```python
from build123d import *

# Parameters (mm, degrees)
SKETCH1_W               = 39.39
SKETCH1_H               = 10
BOSS_EXTRUDE1_DEPTH     = 20
SKETCH2_W               = 31.39
SKETCH2_H               = 10
CUT_EXTRUDE1_DEPTH      = 15
CUT_EXTRUDE2_DEPTH      = 46.294283304
CUT_EXTRUDE2_DEPTH_BACK = 46.294283304
SKETCH3_R               = 1.25
FILLET1_R               = 3
FILLET3_R               = 1
SKETCH4_W               = 20
SKETCH4_H               = 10
BOSS_EXTRUDE2_DEPTH     = 165
FILLET4_R               = 5
SKETCH7_W               = 10
SKETCH7_H               = 10
BOSS_EXTRUDE5_DEPTH     = 2.59
SKETCH8_W               = 10
SKETCH8_H               = 10
BOSS_EXTRUDE6_DEPTH     = 2.59
FILLET7_R               = 3
FILLET11_R              = 3
SKETCH9_R               = 1.25
BOSS_EXTRUDE7_DEPTH     = 10
BOSS_EXTRUDE8_START     = 10
SKETCH10_R              = 1.25
BOSS_EXTRUDE8_DEPTH     = 10


with BuildPart() as part:
    # Sketch1 → Boss-Extrude1 (new body)
    with BuildSketch(Plane.XY):
        with Locations((19.695, 5)):
            Rectangle(SKETCH1_W, SKETCH1_H)
    extrude(amount=BOSS_EXTRUDE1_DEPTH)

    # Sketch2 → Cut-Extrude1 (cut)
    with BuildSketch(Plane.XY.offset(20)):
        with Locations((19.695, 5)):
            Rectangle(SKETCH2_W, SKETCH2_H)
    extrude(amount=-CUT_EXTRUDE1_DEPTH, mode=Mode.SUBTRACT)

    # Sketch3 → Cut-Extrude2 (cut, two sides: drawn at the far end of the back side and taken through both)
    with BuildSketch(Plane.ZY.offset(-CUT_EXTRUDE2_DEPTH_BACK)):
        with Locations(Location((17, 5, 0), (0, 0, 270))):
            Circle(SKETCH3_R)
    extrude(amount=CUT_EXTRUDE2_DEPTH + CUT_EXTRUDE2_DEPTH_BACK, mode=Mode.SUBTRACT)

    # Fillet1
    fillet1_edges = [part.edges().sort_by_distance(p)[0] for p in [
        (4, 5, 5),
        (35.39, 5, 5),
        (39.39, 5, 0),
        (0, 5, 0),
    ]]
    fillet(fillet1_edges, radius=FILLET1_R)

    # Fillet3
    fillet3_edges = [part.edges().sort_by_distance(p)[0] for p in [
        (39.39, 5, 20),
        (4, 5, 20),
        (35.39, 5, 20),
        (0, 5, 20),
    ]]
    fillet(fillet3_edges, radius=FILLET3_R)

    # Sketch4 → Boss-Extrude2 (add)
    with BuildSketch(Plane(origin=(0, 0, 0), x_dir=(-1, 0, 0), z_dir=(0, 0, -1))):
        with Locations((-19.695, 5)):
            Rectangle(SKETCH4_W, SKETCH4_H)
    extrude(amount=BOSS_EXTRUDE2_DEPTH)

    # Fillet4
    fillet4_edges = [part.edges().sort_by_distance(p)[0] for p in [
        (29.695, 5, 0),
        (9.695, 5, 0),
    ]]
    fillet(fillet4_edges, radius=FILLET4_R)

    # Sketch7 → Boss-Extrude5 (add)
    with BuildSketch(Plane.ZY.offset(-9.695)):
        with Locations((-160, 5)):
            Rectangle(SKETCH7_W, SKETCH7_H)
    extrude(amount=BOSS_EXTRUDE5_DEPTH)

    # Sketch8 → Boss-Extrude6 (add)
    with BuildSketch(Plane(origin=(29.695, 0, 0), x_dir=(0, 0, -1), z_dir=(1, 0, 0))):
        with Locations((160, 5)):
            Rectangle(SKETCH8_W, SKETCH8_H)
    extrude(amount=BOSS_EXTRUDE6_DEPTH)

    # Fillet7
    # the kernel refuses this fillet: 3 mm, written as the material it adds along each edge
    with BuildSketch(Plane(origin=(9.695, 0, -155), x_dir=(0, 0, 1), z_dir=(0, 1, 0))) as fillet7_piece_1:
        with BuildLine():
            CenterArc((2.971851275, -3), FILLET7_R, 90, 82.144993797)
            Line((0, -2.59), (-0.059437025, -2.5818))
            ThreePointArc((-0.059437025, -2.5818), (-0.06, -1.295), (-0.06, 0))
            Line((-0.06, 0), (0, 0.06))
            Line((0, 0.06), (2.971851275, 0.06))
            Line((2.971851275, 0.06), (2.971851275, 0))
        make_face()
    extrude(amount=10)
    with BuildSketch(Plane(origin=(29.695, 10, -155), x_dir=(1, 0, 0), z_dir=(0, -1, 0))) as fillet7_piece_2:
        with BuildLine():
            CenterArc((3, 2.971851275), FILLET7_R, 180, 82.144993797)
            Line((0, 2.971851275), (-0.06, 2.971851275))
            Line((-0.06, 2.971851275), (-0.06, 0))
            Line((-0.06, 0), (0, -0.06))
            ThreePointArc((0, -0.06), (1.295, -0.06), (2.5818, -0.059437025))
            Line((2.5818, -0.059437025), (2.59, 0))
        make_face()
    extrude(amount=10)

    # Fillet11
    fillet11_edges = [part.edges().sort_by_distance(p)[0] for p in [
        (19.695, 0, -165),
        (19.695, 10, -165),
    ]]
    fillet(fillet11_edges, radius=FILLET11_R)

    # Sketch9 → Boss-Extrude7 (add)
    with BuildSketch(Plane.ZY.offset(-7.105)):
        with Locations(Location((-162, 5, 0), (0, 0, 180))):
            Circle(SKETCH9_R)
    extrude(amount=BOSS_EXTRUDE7_DEPTH)

    # Sketch10 → Boss-Extrude8 (add)
    with BuildSketch(Plane(origin=(32.285, 0, 0), x_dir=(0, 0, -1), z_dir=(1, 0, 0)).offset(BOSS_EXTRUDE8_START)):
        with Locations((162, 5)):
            Circle(SKETCH10_R)
    extrude(amount=-BOSS_EXTRUDE8_DEPTH)


solid = part.part
```
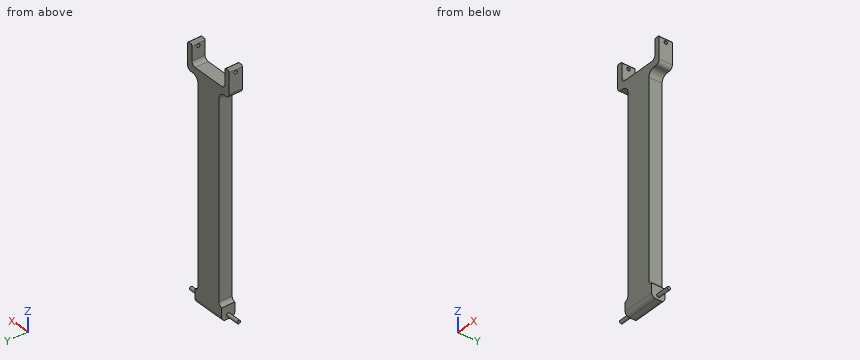
Geometry check sheet. Reference: the model listing, model coordinates, mm. Coordinates: 2 decimals unless noted, no trailing zeros. Order: outer loops, then holes, each group sorted by start corner. A loop starts at its lowest first (then second) coordinate and runs counter-clockwise, first axis right, second up. Notation, with made-up numbers: M -16,-39 L 1,-39 A13 ccw 1,-17 Z; hole C 48,83.5 d9. An arc over 180 degrees is marked long. Answer as a JSON object with one key per item and string values.
Q1. Scan lines: line 1 (Z direction, x = 1.7, y = 5); line 2 (Y direction, x = 38, z = 17); line 3 (X direction, y = 8.75, z = 11). Record each from-to range of solid material in increasing order.
Results are:
{"line 1": "z = -163.25 to -160.75, 0.3 to 15.75, 18.25 to 20", "line 2": "y = 0 to 3.75, 6.25 to 10", "line 3": "x = 0 to 4, 35.39 to 39.39"}
Q2. Depth check by flat-ended pin: pin 1 Ø0.8 at (x, y) = (35.5, 3) entering from -Z; pin 2 Ø1.4 at (x, y) = (3.5, 5) entering from -Z; pin 3 Ø5 at (y, z) = (6, 14.5) entering from -X; pin 4 Ø2 at (y, z) = (5, 17) entering from -X. Enter the tip coordinate at first touch or a pass-through.
Results are:
{"pin 1": "stops at z = 0", "pin 2": "stops at z = -163.25", "pin 3": "stops at x = 0", "pin 4": "passes through"}
Q3. Cross-section at A-A on z = -8.5. Record the cut outline in (x, y) (3 decimals), and give its area (3 significant figures).
Results are:
{"outline": "M 9.695,0 L 29.695,0 L 29.695,10 L 9.695,10 Z", "area": "200 mm²"}
